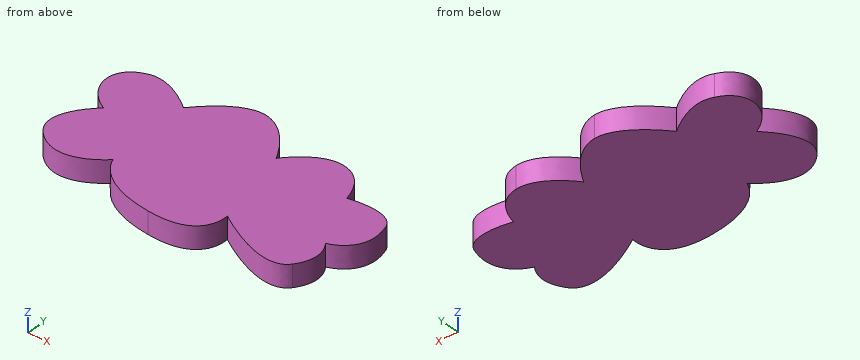
from build123d import *

# Parameters (mm, degrees)
EXTRUDE_DEPTH = 10


with BuildPart() as part:
    # path3336 → Extrude (new body)
    with BuildSketch(Plane(origin=(6.052701, 3.037905, 0), x_dir=(0, -1, 0), z_dir=(0, 0, -1))):
        with BuildLine():
            add(Edge.make_bspline(
                [(-27.698556, 57.875805), (-31.987366, 48.225986), (-20.550543, 34.644759), (-20.550543, 34.644759)],
                knots=[0, 0, 0, 0, 1, 1, 1, 1], degree=3))
            add(Edge.make_bspline(
                [(-20.550543, 34.644759), (-20.550543, 34.644759), (-36.633573, 22.135735), (-35.561372, 10.34151)],
                knots=[0, 0, 0, 0, 1, 1, 1, 1], degree=3))
            add(Edge.make_bspline(
                [(-35.561372, 10.34151), (-34.489167, -1.452715), (-18.048736, -9.315531), (-18.048736, -9.315531)],
                knots=[0, 0, 0, 0, 1, 1, 1, 1], degree=3))
            add(Edge.make_bspline(
                [(-18.048736, -9.315531), (-18.048736, -9.315531), (-31.272565, -18.965352), (-29.84296, -30.044777)],
                knots=[0, 0, 0, 0, 1, 1, 1, 1], degree=3))
            add(Edge.make_bspline(
                [(-29.84296, -30.044777), (-28.413357, -41.124198), (-15.546932, -43.268601), (-15.546932, -43.268601)],
                knots=[0, 0, 0, 0, 1, 1, 1, 1], degree=3))
            add(Edge.make_bspline(
                [(-15.546932, -43.268601), (-15.546932, -43.268601), (-20.27429, -61.656045), (-10.900722, -64.712644)],
                knots=[0, 0, 0, 0, 1, 1, 1, 1], degree=3))
            add(Edge.make_bspline(
                [(-10.900722, -64.712644), (5.53971, -70.073653), (9.82852, -55.062826), (9.82852, -55.062826)],
                knots=[0, 0, 0, 0, 1, 1, 1, 1], degree=3))
            add(Edge.make_bspline(
                [(9.82852, -55.062826), (9.82852, -55.062826), (16.976534, -61.496036), (26.626353, -54.348025)],
                knots=[0, 0, 0, 0, 1, 1, 1, 1], degree=3))
            add(Edge.make_bspline(
                [(26.626353, -54.348025), (37.524521, -46.275309), (19.120938, -18.607952), (19.120938, -18.607952)],
                knots=[0, 0, 0, 0, 1, 1, 1, 1], degree=3))
            add(Edge.make_bspline(
                [(19.120938, -18.607952), (19.120938, -18.607952), (36.633573, -21.467156), (34.489167, 4.265697)],
                knots=[0, 0, 0, 0, 1, 1, 1, 1], degree=3))
            add(Edge.make_bspline(
                [(34.489167, 4.265697), (32.344764, 29.99855), (18.763534, 33.215156), (18.763534, 33.215156)],
                knots=[0, 0, 0, 0, 1, 1, 1, 1], degree=3))
            add(Edge.make_bspline(
                [(18.763534, 33.215156), (18.763534, 33.215156), (35.36464, 48.774395), (21.980142, 62.164612)],
                knots=[0, 0, 0, 0, 1, 1, 1, 1], degree=3))
            add(Edge.make_bspline(
                [(21.980142, 62.164612), (11.904058, 72.245005), (-2.680508, 55.731399), (-2.680508, 55.731399)],
                knots=[0, 0, 0, 0, 1, 1, 1, 1], degree=3))
            add(Edge.make_bspline(
                [(-2.680508, 55.731399), (-9.214777, 68.682765), (-23.253633, 70.123036), (-27.698556, 57.875805)],
                knots=[0, 0, 0, 0, 1, 1, 1, 1], degree=3))
        make_face()
    extrude(amount=-EXTRUDE_DEPTH)


solid = part.part
The listing builds one solid part. Answer for the finished solid, in the listing's coordinates (mm). Give positions to 0.01 mm unless a question says otherwise; leave off trailing zeros. One line per item, written item: value. Start each with the question number.
1) Given pin 1 Ø1 at (y, z) = (29, 8.5) entering from +X; pin 2 Ø3 at (x, z) = (-18.5, 2) entering from -Y; pin 3 Ø1.5 at (y, z) = (-15, 1) entering from -X, each flat-ended and moving along its own axis, determine where each tip first touches the part or whether it passes through.
2) A cutting plane is placed at A-A on y = 25. State how many separate pieces and enclosed holes the cut face has, then the cut area to 3 significant figures.
3) Find the intervals of material crossed by L1, parallel to X at y = -18.5, z = 1.25; L2, parallel to X at y = -15, z = 9.25; L3, parallel to Y at x = -6, z = 9.25, in increasing order.
Answer sheet:
1. pin 1: stops at x = 44.49
1. pin 2: stops at y = -26.5
1. pin 3: stops at x = -58.98
2. separate pieces: 3
2. enclosed holes: 0
2. area: 973 mm2
3. L1: x = -56.53 to -30.29, -25.91 to 24.73, 28.61 to 63.11
3. L2: x = -58.73 to 63.76
3. L3: y = -30.34 to 38.64
